Build history of the part. All positions in model axes, mm. A direction names the side the tool comes from. Round coordinates to 2 decimals unless told otherwise and drop trailing zeros. Write each loop counter-clockwise with the first axis right and the second up, starting at its lowest first coordinate (ties: lowest second). Pieces come first, ordered by that corner, then holes.
1) Saw through at A-A (x = -24.15). Write the cut outline in (y, z).
2) Saw through at C-C (z = 25.5). Write the cut outline in (x, y), plus the area to 3 significant figures.
3) Flat gauge pins, fed straight in: pin 1 (5.5 mm diameter, centred on x = 24.15, y = 5.65, fed in from -Z); pin 2 (5 mm diameter, centred on x = -13, y = 3.5, fed in from +Z); pin 3 (3.5 mm diameter, centred on x = 23, y = 4, fed in from -Z). Where does each tip first touch, or does it go through?
4) Saw through at B-B (x = 24). State how many separate pieces and enclosed holes the cut face has, plus the area to 3 significant figures.
5) Wall check: probe 1 along Y at (x, z) = (24, 30); probe 2 along Y at (x, z) = (23, 31); probe 3 along X at (y, z) = (-7.5, 33). Give the ranges that are in metal, low to high.
6) Which spindle directions (+Z, -Z, +X, -X, +Y, -Y) get a long thin tool onto all of the face, cutting with end or side? Do faces 1 (the flat face through (-20.45, 0, 14)), 2 (the flat face through (-27, 4.425, 30)), 3 (the flat face through (20.45, 0, 34)). Say none if no direction does.
7) Pull direction Y, two halves, no side cores. Call faces 4 (the cylindrical face through (13.226, 0.874, 42.522)), 5 (the flat face through (27, -4.425, 30)), 6 (the flat face through (18, -8, 36.7)), 7 (the flat face through (27, 4.425, 30)): +Y half, -Y half, draft (parallel to the pull), parting line (faces both ways), or undercut.
from build123d import *

# Parameters (mm, degrees)
SKETCH_1_W             = 40.9
SKETCH_1_H             = 20
EXTRUDE_1_DEPTH        = 36.7
SKETCH_2_R             = 10
EXTRUDE_2_DEPTH        = 2
SKETCH_3_R             = 6.54
EXTRUDE_3_DEPTH        = 1.3
SKETCH_4_R             = 5.35
EXTRUDE_4_DEPTH        = 0.55
SKETCH_5_R             = 2.91
SKETCH_5_R_2           = 1.275
EXTRUDE_5_DEPTH        = 4
EXTRUDE_6_DEPTH        = 2
SKETCH_7_W             = 2.52
SKETCH_7_H             = 20
EXTRUDE_7_DEPTH        = 7.4
CUT_EXTRUDE_3_DEPTH    = 3.4
FILLET_1_R             = 1
FILLET_1_OF_MIRROR_1_R = 1
SKETCH_9_W             = 4.1
SKETCH_9_H             = 7.35
EXTRUDE_8_DEPTH        = 5.2
EXTRUDE_8_TAPER        = 8


with BuildPart() as part:
    # 스케치1 → 보스-돌출1 (new body)
    with BuildSketch(Plane.XY):
        Rectangle(SKETCH_1_W, SKETCH_1_H)
    extrude(amount=EXTRUDE_1_DEPTH)

    # 스케치2 → 보스-돌출2 (add)
    with BuildSketch(Plane.XY.offset(36.7)):
        with Locations((10.45, 0)):
            Circle(SKETCH_2_R)
    extrude(amount=EXTRUDE_2_DEPTH)

    # 스케치3 → 보스-돌출3 (add)
    with BuildSketch(Plane.XY.offset(38.7)):
        with Locations((10.45, 0)):
            Circle(SKETCH_3_R)
    extrude(amount=EXTRUDE_3_DEPTH)

    # 스케치4 → 보스-돌출4 (add)
    with BuildSketch(Plane.XY.offset(40)):
        with Locations((10.45, 0)):
            Circle(SKETCH_4_R)
    extrude(amount=EXTRUDE_4_DEPTH)

    # 스케치5 → 보스-돌출5 (add)
    with BuildSketch(Plane.XY.offset(40.55)):
        with Locations((10.45, 0)):
            Circle(SKETCH_5_R)
        with Locations((10.45, 0)):
            Circle(SKETCH_5_R_2, mode=Mode.SUBTRACT)
    extrude(amount=EXTRUDE_5_DEPTH)

    # 스케치6 → 보스-돌출6 (add)
    with BuildSketch(Plane.XY.offset(36.7)):
        with BuildLine():
            Line((5.939526078, 8.925), (-14.6, 8.925))
            Line((-14.6, 8.925), (-14.6, -8.925))
            Line((-14.6, -8.925), (5.939526078, -8.925))
            ThreePointArc((5.939526078, -8.925), (0.45, 0), (5.939526078, 8.925))
        make_face()
    extrude(amount=EXTRUDE_6_DEPTH)

    # 스케치7 → 보스-돌출7 (add)
    with BuildSketch(Plane(origin=(20.45, 0, 0), x_dir=(0, 0, -1), z_dir=(1, 0, 0))):
        with Locations((-29.96, 0)):
            Rectangle(SKETCH_7_W, SKETCH_7_H)
    extrude_7 = extrude(amount=EXTRUDE_7_DEPTH)

    # 스케치8 → 컷-돌출3 (cut)
    with BuildSketch(Plane.XY.offset(31.22)):
        with BuildLine():
            Line((27.85, 6.875), (27.85, 4.425))
            Line((27.85, 4.425), (25.977395688, 4.425))
            ThreePointArc((25.977395688, 4.425), (21.95, 5.65), (25.977395688, 6.875))
            Line((25.977395688, 6.875), (27.85, 6.875))
        make_face()
        with BuildLine():
            Line((27.85, -4.425), (27.85, -6.875))
            Line((27.85, -6.875), (25.977395688, -6.875))
            ThreePointArc((25.977395688, -6.875), (21.95, -5.65), (25.977395688, -4.425))
            Line((25.977395688, -4.425), (27.85, -4.425))
        make_face()
    cut_extrude_3 = extrude(amount=-CUT_EXTRUDE_3_DEPTH, mode=Mode.SUBTRACT)

    # 필렛1
    fillet_1_edges = [part.edges().sort_by_distance(p)[0] for p in [
        (27.85, -10, 29.96),
        (27.85, 10, 29.96),
    ]]
    fillet(fillet_1_edges, radius=FILLET_1_R)

    # 대칭 복사1: 보스-돌출7, 컷-돌출3 across plane
    add(extrude_7.mirror(Plane(origin=(0, 0, 0), x_dir=(0, 0, 1), z_dir=(1, 0, 0))))
    add(cut_extrude_3.mirror(Plane(origin=(0, 0, 0), x_dir=(0, 0, 1), z_dir=(1, 0, 0))), mode=Mode.SUBTRACT)

    # 필렛1 of 대칭 복사1
    fillet_1_of_mirror_1_edges = [part.edges().sort_by_distance(p)[0] for p in [
        (-27.85, -10, 29.96),
        (-27.85, 10, 29.96),
    ]]
    fillet(fillet_1_of_mirror_1_edges, radius=FILLET_1_OF_MIRROR_1_R)

    # 스케치9 → 보스-돌출8 (add)
    with BuildSketch(Plane(origin=(20.45, 0, 0), x_dir=(0, 0, -1), z_dir=(1, 0, 0))):
        with Locations((-6.23, 0)):
            Rectangle(SKETCH_9_W, SKETCH_9_H)
    extrude(amount=EXTRUDE_8_DEPTH, taper=EXTRUDE_8_TAPER)


solid = part.part
Evaluation:
1. outline: (-10, 28.7) - (-7.85, 28.7) - (-7.85, 31.22) - (-10, 31.22) - close; (-3.45, 28.7) - (3.45, 28.7) - (3.45, 31.22) - (-3.45, 31.22) - close; (7.85, 28.7) - (10, 28.7) - (10, 31.22) - (7.85, 31.22) - close
2. outline: (-20.45, -10) - (20.45, -10) - (20.45, 10) - (-20.45, 10) - close
2. area: 818 mm2
3. pin 1: stops at z = 4.48
3. pin 2: stops at z = 38.7
3. pin 3: stops at z = 4.3
4. separate pieces: 4
4. enclosed holes: 0
4. area: 48.0 mm2
5. probe 1: y = -10 to -7.84, -3.46 to 3.46, 7.84 to 10
5. probe 2: y = -10 to -7.53, -3.77 to 3.77, 7.53 to 10
5. probe 3: x = -20.45 to 20.45
6. face 1: -Z, -X, +Y, -Y
6. face 2: +Z, -Z, -X
6. face 3: +Z, +X, +Y, -Y
7. face 4: parting line
7. face 5: undercut
7. face 6: draft
7. face 7: undercut
